Read the model definition and answer for the solid it produces. Units are mm, in the model's axes. Face numbers are marked on the shaded views. A direction names the side the tool comes from. Give positions to 0.01 mm unless a question says otherwise; leave off trailing zeros. Write each loop counter-clockwise with the first axis right and the second up, starting at its lowest first coordinate (ties: lowest second). Pieces come first, ordered by that corner, then holes. Notation, with made-up numbers: M -31,54 L 10,54 A30 ccw 10,84 Z; hole C -34.5,-5.75 d6. An arc over 180 degrees is marked long. Put each result on its own line as item: value.
from build123d import *

# Parameters (mm, degrees)
SKETCH_1_R      = 1.5
EXTRUDE_1_DEPTH = 6
SKETCH_2_R      = 2.85
EXTRUDE_2_DEPTH = 1.65
FILLET_1_R      = 2


with BuildPart() as part:
    # 草图1 → 凸台-拉伸1 (new body)
    with BuildSketch(Plane.XY):
        Circle(SKETCH_1_R)
    extrude(amount=EXTRUDE_1_DEPTH)

    # 草图2 → 凸台-拉伸2 (add)
    with BuildSketch(Plane(origin=(0, 0, 0), x_dir=(-1, 0, 0), z_dir=(0, 0, -1))):
        Circle(SKETCH_2_R)
    extrude(amount=EXTRUDE_2_DEPTH)

    # 圆角1
    # the kernel refuses this fillet: 2 mm, written as the material it takes off along each edge
    with BuildSketch(Plane(origin=(0, 0, -1.65), x_dir=(-1, 0, 0), z_dir=(0, -1, 0))) as fillet_1_piece_1:
        with BuildLine():
            CenterArc((0.880863133, -2), FILLET_1_R, 10.078658108, 79.921341892)
            Line((0.880863133, 0), (0.880863133, 0.04))
            Line((0.880863133, 0.04), (2.85, 0.04))
            Line((2.85, 0.04), (2.89, 0))
            ThreePointArc((2.89, 0), (2.89, -0.825), (2.889382737, -1.643))
            Line((2.889382737, -1.643), (2.85, -1.65))
        make_face()
    revolve(axis=Axis((0, 0, -1.65), (0, 0, -1)), mode=Mode.SUBTRACT)


solid = part.part
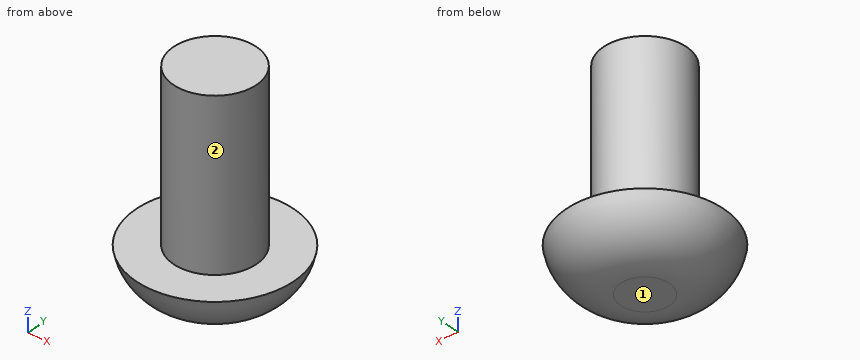
(1) Given pin 1 Ø1 at (y, z) = (-2, 0) entering from -X; pin 2 Ø2 at (x, z) = (-2, 5) entering from -Y, each flat-ended and moving along its own axis, determine where each tip first touches the part or whether it passes through.
Result:
pin 1: stops at x = -2.42
pin 2: stops at y = -1.12
(2) Section A-A on z = 3.25 is taken. Determine the outline of the cut face in (x, y), and give its area (3 significant figures).
Result:
outline: C 0,0 d3
area: 7.07 mm²
(3) Straight lines are drawn through the part: line 1 along X through (y, z) = (1.05, 5.75); line 2 along X through (y, z) = (0.35, 5.25); line 3 along Y through (x, z) = (1.25, 0.75). For each, find the intervals that lie inside material, in ascending order. Write a range as from..to.
Result:
line 1: x = -1.07..1.07
line 2: x = -1.46..1.46
line 3: y = -0.83..0.83
(4) Which of the six approach directions +Z, -Z, +X, -X, +Y, -Y give full straight-line access (tool end or side, diameter ignored) to the marked faces 1 and 2?
Result:
face 1: -Z, +X, -X, +Y, -Y
face 2: +Z
